Autodesk Fusion 360 part; units mm, degrees
sketch "Sketch1" plane through (0, 0, 0) normal (0, 0, 1) x (1, 0, 0)
  line L0 (0, 0) -> (113.5, 0)
  line L1 (113.5, 0) -> (113.5, 69.5)
  line L2 (113.5, 69.5) -> (0, 69.5)
  line L3 (0, 69.5) -> (0, 0)
  line L4 (56.75, 69.5) -> (56.75, 0) construction
  line L5 (0, 34.75) -> (113.5, 34.75) construction
  line L6 (-10.75, 74.2) -> (124.25, 74.2)
  line L7 (124.25, 74.2) -> (124.25, -4.7)
  line L8 (124.25, -4.7) -> (-10.75, -4.7)
  line L9 (-10.75, -4.7) -> (-10.75, 74.2)
  line L10 (56.75, 74.2) -> (56.75, -4.7) construction
  line L11 (-10.75, 34.75) -> (124.25, 34.75) construction
  circle A0 centre (-4.75, 68.2) radius 1.1
  circle A1 centre (-4.75, 1.3) radius 1.1
  circle A2 centre (118.25, 1.3) radius 1.1
  circle A3 centre (118.25, 68.2) radius 1.1
  dimension "d1" = 113.5
  dimension "d2" = 69.5
  dimension "d3" = 78.9
  dimension "d4" = 135
  dimension "d5" = 2.2
  dimension "d6" = 2.2
  dimension "d7" = 2.2
  dimension "d8" = 2.2
  dimension "d9" = 6
  dimension "d10" = 6
  dimension "d11" = 6
  dimension "d12" = 6
  dimension "d13" = 6
  dimension "d14" = 6
  dimension "d15" = 6
  dimension "d16" = 6
extrude "Extrude1" add sketch "Sketch1" against normal blind 30 contours L6 L7 L8 L9 | A0 | A1 | A2 | A3
sketch "Sketch2" plane through (124.25, 0, 0) normal (1, 0, 0) x (0, 1, 0)
  line L0 (74.2, 0) -> (-4.7, 0)
  line L1 (-4.7, 0) -> (-4.7, -30)
  line L2 (-4.7, -30) -> (74.2, -30)
  line L3 (74.2, -30) -> (74.2, 0)
  line L4 (-26.2609, 0) -> (74.2, 0)
  line L5 (-26.2609, 0) -> (8.4215, -95.2891)
  line L6 (8.4215, -95.2891) -> (74.2, -71.3477)
  line L7 (74.2, -71.3477) -> (74.2, 0)
  line L8 (-15.6191, 0) -> (17.8184, -91.8689)
  line L9 (-4.7, 0) -> (-4.7, -30)
  line L10 (69.5, 0) -> (69.5, -73.0584)
  point P0 (69.5, -30)
  point P1 (0, -30)
  dimension "d19" = 70
  dimension "d20" = 10
  dimension "d21" = 70
  dimension "d22" = 90
extrude "Extrude2" add sketch "Sketch2" against normal blind 135 contours L2 L6 L7 L10 | L1 L4 L8 L9 | L4 L5 L6 L8
extrude "Extrude3" add sketch "Sketch2" against normal blind 10.75 contours L2 L6 L8 L10
extrude "Extrude4" add sketch "Sketch2" along normal blind 10.75 from surface at -135 contours L2 L6 L8 L10
chamfer "Chamfer1" distance 4.7 angle 45 1 edges at (56.75, -4.7, -30)
extrude "Extrude5" cut sketch "Sketch1" against normal blind 10 contours A0 | A1 | A2 | A3
fillet "Fillet1" radius 6 2 edges at (124.25, 74.2, -35.6739) (-10.75, 74.2, -35.6739)
Part model, mm, in its own coordinate system. A direction names the side the tool comes from. Round coordinates to 2 decimals unless told otherwise and drop trailing zeros. Write each loop counter-clockwise with the first axis right and the second up, starting at its lowest first coordinate (ties: lowest second). Pieces come first, ordered by that corner, then holes. Notation, with made-up numbers: M 10,65 L 47,65 A10 ccw 47,69 Z; hole C 86.25,-3 d5. An arc over 180 degrees is marked long. Return JSON: item names as keys, results as strings. Group by question number.
(1) Saw through at A-A on y = 44. Write the cut outline in (x, z).
(2) Which spindle directions (+Z, -Z, +X, -X, +Y, -Y) get a long thin tool onto all of the face, cutting with end or side? Do faces 1 (the face through (58, 69.5, -36)), 2 (the face through (-10.75, 31, -36)), 3 (the face through (56, 0, -15)). Say none if no direction does.
(3) Saw through at B-B on z = -44.5. Write the cut outline in (x, y).
(4) Pin check, flat tips, straight feed: pin 1 Ø5 at (x, z) = (50, -67.5) entering from -Y; pin 2 Ø8 at (x, z) = (24, -65.5) entering from -Y; pin 3 Ø2.5 at (x, y) = (118.25, 68.2) entering from -Z. Stop position of each tip, or through.
(5) Saw through at D-D on y = 11. Write the cut outline in (x, z).
(6) Drill centre lines: probe 1 along X at (y, z) = (68.2, -5.75); probe 2 along X at (y, z) = (68, -2); probe 3 along X at (y, z) = (6.5, -5). Where is each one in solid material? Low to high.
(7) Two-plate mould, pull along Y, no slides. Class faces 4 (the face through (57.7, -9.16, -46.98)), 5 (the face through (56, 74.2, -35)), 6 (the face through (55.956, -1.525, -32.177)), 7 (the face through (113.5, 33, -35)): +Y half, -Y half, draft (parallel to the pull), parting line (faces both ways), or undercut.
Returned:
{
 "1": {"outline": "M -10.75,-82.34 L 0,-82.34 L 0,0 L -10.75,0 Z; M 113.5,-82.34 L 124.25,-82.34 L 124.25,0 L 113.5,0 Z"},
 "2": {"face 1": "+Z, -Z", "face 2": "+Z, -Z, -X, +Y, -Y", "face 3": "+Z"},
 "3": {"outline": "M -10.75,-10.06 L 124.25,-10.06 L 124.25,68.2 A6 ccw 118.25,74.2 L -4.75,74.2 A6 ccw -10.75,68.2 Z; hole M 0,0.58 L 113.5,0.58 L 113.5,69.5 L 0,69.5 Z"},
 "4": {"pin 1": "y = -2.6", "pin 2": "y = -3.88", "pin 3": "z = -73.99"},
 "5": {"outline": "M -10.75,-94.35 L 124.25,-94.35 L 124.25,0 L 113.5,0 L 113.5,-73.14 L 0,-73.14 L 0,0 L -10.75,0 Z"},
 "6": {"probe 1": "-10.75 to -5.85, -3.65 to 0, 113.5 to 117.15, 119.35 to 124.25", "probe 2": "-10.75 to -5.83, -3.67 to 0, 113.5 to 117.17, 119.33 to 124.25", "probe 3": "-10.75 to 0, 113.5 to 124.25"},
 "7": {"face 4": "-Y half", "face 5": "+Y half", "face 6": "undercut", "face 7": "undercut"}
}
